Read the model definition and answer for the solid it produces. Units are mm, in the model's axes. A direction names the side the tool comes from. Coordinates: 2 decimals unless noted, no trailing zeros. Write each loop counter-clockwise with the first axis right and the second up, starting at its lowest first coordinate (ties: lowest second). Pieces come first, ordered by that corner, then holes. Notation, with made-up numbers: (14.25, 41) -> (73.25, 41) arc R26 ccw to (73.25, 64) -> close; hole circle Ø1 at (72.5, 75.25). An arc over 180 degrees is marked (long way). Answer as a JSON object with one key per item and string values. Group by question number.
(1) Flat-ended cylindrical pins translate along their axes: P1, Ø1, axis at x = -9, z = 4.5, coming from the -Y side; P2, Ø4, axis at y = 0, z = -52.5, coming from the -X side; P3, Ø5, axis at y = -9.5, z = 31, coming from the -X side; P4, Ø6, axis at x = -16, y = 2, coming from the -Z side. Find the tip coordinate at first contact, or state that the pin passes through.
(2) For a pull along Y with two mould halves and no side action, classify faces 1 (the face through (21.938, -6.909, -1.155)), 2 (the face through (-7, 19, -82.5)), 3 (the face through (19.076, -6.007, -1.155)) as +Y half, -Y half, draft (parallel to the pull), parting line (faces both ways), or undercut.
(3) Find section B-B (y = -6). Give the vertices of the cut face in (x, z), then the cut area to 3 significant figures.
(4) Find section D-D (z = 52.5). Give the vertices of the cut face in (x, y), then the cut area to 3 significant figures.
(5) Find section C-C (z = 73.5). Give the vertices of the cut face in (x, y).
(6) Which of the six approach directions +Z, -Z, +X, -X, +Y, -Y give full straight-line access (tool end or side, diameter ignored) to faces 4 (the face through (-7, 19, 82.5)), 5 (the face through (-21.459, -0.099, -50.252))?
(7) Straight lines are drawn through the part: L1, parallel to Y at x = 0, z = -21; L2, parallel to Y at x = 15, z = -11.5; L3, parallel to X at y = -4, z = -50.5. For each, find the intervals that lie inside material, in ascending order.
(8) Find section A-A (x = 0). Give the vertices of the cut face in (y, z), then the cut area to 3 significant figures.
Autodesk Inventor part; units mm, degrees
ref_plane "YZ Plane" through (0, 0, 0) normal (1, 0, 0) x (0, 1, 0)
ref_plane "XZ Plane" through (0, 0, 0) normal (0, 1, 0) x (-1, 0, 0)
ref_plane "XY Plane" through (0, 0, 0) normal (0, 0, 1) x (1, 0, 0)
sketch "Sketch1" plane through (0, 0, 0) normal (0, 0, 1) x (1, 0, 0)
  circle A0 centre (0, 0) radius 20
  circle A1 centre (0, 0) radius 23
  dimension "d0" = 40
  dimension "d1" = 46
extrude "Extrusion1" add sketch "Sketch1" along normal mid plane 165
sketch "Sketch2" plane through (0, 0, 0) normal (1, 0, 0) x (0, 1, 0)
  line L0 (0, 35) -> (0, -35)
  line L1 (-32.2, 0) -> (32.2, 0)
  line L2 (23, 82.5) -> (-23, 82.5)
  line L3 (-23, -82.5) -> (23, -82.5)
  line L4 (20, -82.5) -> (-20, -82.5)
  point P0 (0, 0)
  point P1 (0, 52.5)
  point P2 (0, -52.5)
  point P3 (0, -82.5)
  dimension "d21" = 105
  dimension "d22" = 30
  dimension "d24" = 30
hole "Hole1" at (0, 0, 52.5) at (0, 0, -52.5) direction (-1, 0, 0) diameter 4.5 end through all
sketch "Sketch3" plane through (0, 0, 0) normal (1, 0, 0) x (0, 1, 0)
  line L0 (23, -82.5) -> (7, -82.5)
  line L1 (7, -82.5) -> (7, 82.5)
  line L2 (7, 82.5) -> (23, 82.5)
  line L3 (23, 82.5) -> (23, -82.5)
  line L4 (23, 82.5) -> (-23, 82.5)
  line L5 (-23, -82.5) -> (23, -82.5)
  line L6 (0, 35) -> (0, -35)
  point P0 (0, 0)
  dimension "d13" = 0
  dimension "d14" = 0
  dimension "d15" = 7
extrude "Extrusion2" [suppressed]
properties part number "Top_Separator Pipe Long" material "PVC-Piping"
Results below:
{
 "1": {"P1": "stops at y = -21.37", "P2": "stops at x = 19.9", "P3": "stops at x = -21.91", "P4": "passes through"},
 "2": {"face 1": "parting line", "face 2": "draft", "face 3": "undercut"},
 "3": {"outline": "(-22.2, -82.5) -> (-19.08, -82.5) -> (-19.08, 82.5) -> (-22.2, 82.5) -> close; (19.08, -82.5) -> (22.2, -82.5) -> (22.2, 82.5) -> (19.08, 82.5) -> close", "area": "1,030 mm2"},
 "4": {"outline": "(-22.89, -2.25) arc R23 ccw (long way) to (-22.89, 2.25) -> (-19.87, 2.25) arc R20 cw (long way) to (-19.87, -2.25) -> close", "area": "392 mm2"},
 "5": {"outline": "circle Ø46 at (0, 0); hole circle Ø40 at (0, 0)"},
 "6": {"face 4": "+Z, +X, -X, +Y, -Y", "face 5": "-X"},
 "7": {"L1": "y = -23 to -20, 20 to 23", "L2": "y = -17.44 to -13.23, 13.23 to 17.44", "L3": "x = -22.65 to -19.6, 19.6 to 22.65"},
 "8": {"outline": "(-23, -82.5) -> (-20, -82.5) -> (-20, 82.5) -> (-23, 82.5) -> close; (20, -82.5) -> (23, -82.5) -> (23, 82.5) -> (20, 82.5) -> close", "area": "990 mm2"}
}
